Part model, mm, in its own coordinate system. A direction names the side the tool comes from. Round coordinates to 2 decimals unless told otherwise and drop trailing zeros. Order: outer loops, then holes, each group sorted by start corner. A loop starts at its lowest first (then second) coordinate and runs counter-clockwise, first axis right, second up. Notation, with made-up numbers: M -27.75,-34.75 L 13.25,-34.75 A38 cw 13.25,3.25 Z; hole C 72,-35.5 d7. An arc over 180 degrees is marked long. One line per question, with ' | ' between items.
Autodesk Inventor part; units mm, degrees
ref_plane "YZ Plane" through (0, 0, 0) normal (1, 0, 0) x (0, 1, 0)
ref_plane "XZ Plane" through (0, 0, 0) normal (0, 1, 0) x (-1, 0, 0)
ref_plane "XY Plane" through (0, 0, 0) normal (0, 0, 1) x (1, 0, 0)
sketch "Sketch1" plane through (0, 0, 0) normal (0, 0, 1) x (1, 0, 0)
  line L0 (0, 21) -> (0, 6)
  line L1 (0, 0) -> (35, 0) construction
  line L2 (35, 0) -> (35, 6) construction
  line L3 (35, 10) -> (8, 10)
  line L4 (8, 10) -> (8, 21)
  line L5 (8, 21) -> (0, 21)
  line L6 (35, 6) -> (0, 6)
  line L7 (0, 6) -> (0, 0) construction
  line L8 (35, 6) -> (35, 10)
  dimension "d0" = 10
  dimension "d1" = 21
  dimension "d2" = 8
  dimension "d3" = 35
  dimension "d4" = 6
revolve "Revolution1" add sketch "Sketch1" angle 360 about axis through (0, 0, 0) along (1, 0, 0)
sketch "Sketch2" plane through (0, 0, 0) normal (-1, 0, 0) x (0, 0, 1)
  circle A0 centre (0, 0) radius 21
  circle A1 centre (0, 0) radius 21
  line L0 (-14.8492, 14.8492) -> (-14.8492, -14.8492)
  line L1 (14.8492, -14.8492) -> (14.8492, 14.8492)
  line L2 (0, 0) -> (14.8492, 14.8492) construction
  circle A2 centre (0, 16) radius 2.4
  circle A3 centre (11.3137, 11.3137) radius 2.4
  circle A4 centre (11.3137, -11.3137) radius 2.4
  circle A5 centre (0, 0) radius 16 construction
  circle A6 centre (-11.3137, 11.3137) radius 2.4
  circle A7 centre (0, -16) radius 2.4
  circle A8 centre (-11.3137, -11.3137) radius 2.4
  point P0 (-14.8492, -14.8492)
  dimension "d6" = 45
  dimension "d7" = 32
  dimension "d8" = 4.8
extrude "Extrusion1" cut sketch "Sketch2" against normal blind 10 contours A0 L1 | L0 A0 | A2 | A3 | A4 | A6 | A7 | A8
properties part number "SFU1204-Housing"
1) Saw through at D-D (y = 12.5). List the corners of the cut face in (x, z), plus the area to 3 significant figures.
The answers:
outline: M 0,-14.85 L 8,-14.85 L 8,-13.4 L 0,-13.4 Z; M 0,-9.23 L 8,-9.23 L 8,9.23 L 0,9.23 Z; M 0,13.4 L 8,13.4 L 8,14.85 L 0,14.85 Z | area: 171 mm²
2) Saw through at B-B (y = 0). List the corners of the cut face in (x, z), plus the area to 3 significant figures.
The answers:
outline: M 0,-14.85 L 8,-14.85 L 8,-10 L 35,-10 L 35,-6 L 0,-6 Z; M 0,6 L 35,6 L 35,10 L 8,10 L 8,14.85 L 0,14.85 Z | area: 358 mm²
3) Two-plate mould, pull along Z, no slides. Class faces 3 (the face through (21.31, -2.17, 9.76)), 4 (the face through (0, -5, 4)), 5 (the face through (3.944, -10.593, -9.025)), 6 (the face through (17, -6, 0)): released by +Z, released by -Z, zero draft, split by the parting line, or undercut.
The answers:
face 3: split by the parting line | face 4: zero draft | face 5: undercut | face 6: undercut
4) Probe line 1 (Y direction, x = 2, z = 11.25); line 2 (Y direction, x = 4, z = -5); line 3 (X direction, y = 19, z = -4). List the from-to ranges inside material, lowest first. Write a range as [from, to].
The answers:
line 1: y = [-17.73, -13.71], [-8.91, 8.91], [13.71, 17.73] | line 2: y = [-20.4, -3.32], [3.32, 20.4] | line 3: x = [0, 8]
5) Which spindle directions (+Z, -Z, +X, -X, +Y, -Y) get a long thin tool onto all of the face, cutting with end or side? Do faces 1 (the face through (4, 0, -14.849)), 2 (the face through (8, 4, 10)). Say none if no direction does.
The answers:
face 1: -Z, +X, -X, +Y, -Y | face 2: +X
6) Saw through at A-A (z = 0). List the corners of the cut face in (x, y), plus the area to 3 significant figures.
The answers:
outline: M 0,-21 L 8,-21 L 8,-18.4 L 0,-18.4 Z; M 0,-13.6 L 8,-13.6 L 8,-10 L 35,-10 L 35,-6 L 0,-6 Z; M 0,6 L 35,6 L 35,10 L 8,10 L 8,13.6 L 0,13.6 Z; M 0,18.4 L 8,18.4 L 8,21 L 0,21 Z | area: 379 mm²
7) Saw through at C-C (z = -10.75). List the corners of the cut face in (x, y), plus the area to 3 significant figures.
The answers:
outline: M 0,-18.04 L 8,-18.04 L 8,-13.65 L 0,-13.65 Z; M 0,-8.98 L 8,-8.98 L 8,8.98 L 0,8.98 Z; M 0,13.65 L 8,13.65 L 8,18.04 L 0,18.04 Z | area: 214 mm²
8) Drop flat-ended pins along their axis: pin 1 (1.5 mm diameter, centred on y = -5, z = -2.5, fed in from -X); pin 2 (8 mm diameter, centred on x = 30, z = 0.5, fed in from -Y); pin 3 (12 mm diameter, centred on x = 22, z = 10.5, fed in from -Y); pin 4 (6 mm diameter, centred on x = 28, z = 1, fed in from +Y). Give the stop position or say it passes through.
The answers:
pin 1: stops at x = 0 | pin 2: stops at y = -10 | pin 3: stops at y = -8.93 | pin 4: stops at y = 10
